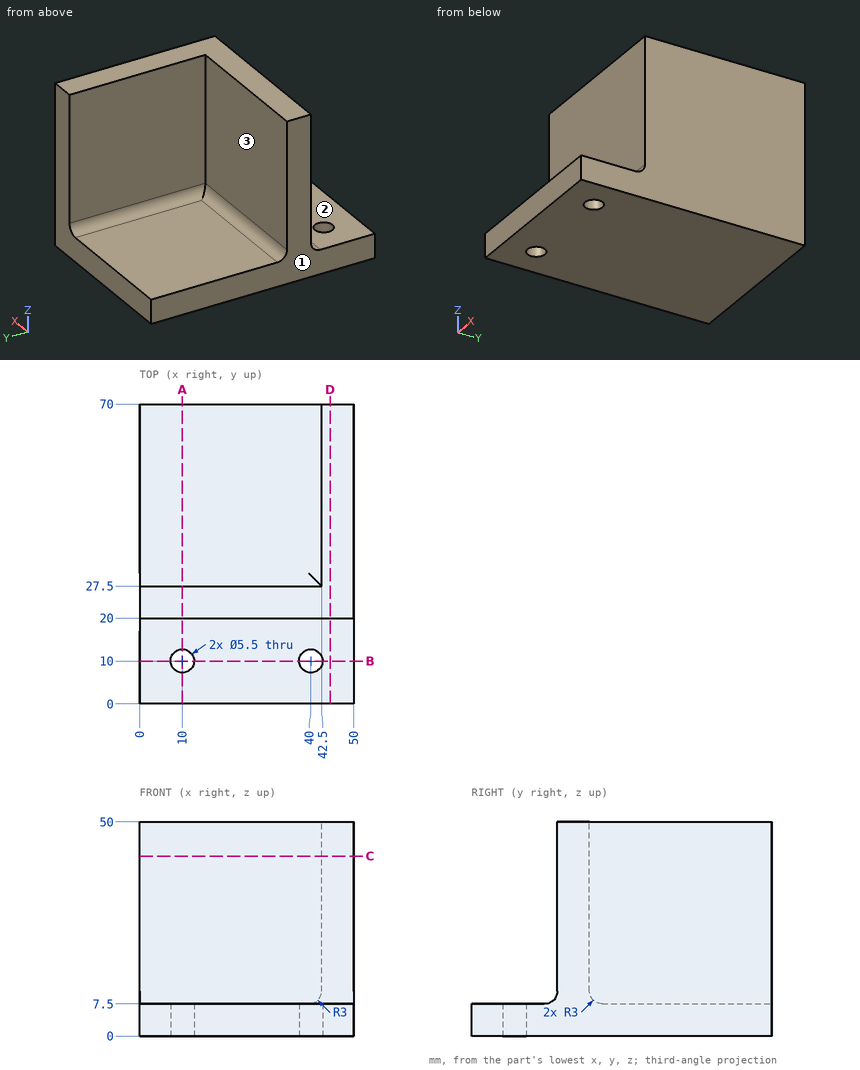
Geometry check sheet. Reference: drawing and pictorial views, mm from the part's lowest x, y, z. A direction names the side the tool comes from. Give positions to 0.01 mm unless a question says otherwise; leave off trailing zeros. Write each loop counter-clockwise with the first axis right and the second up, starting at its lowest first coordinate (ties: lowest second). Pieces come first, ordered by that corner, then holes. Notation, with made-up numbers: M 20.25,-3 L 75.25,-3 A5 cw 75.25,3 Z; hole C -2,59.25 d8. An arc over 180 degrees is marked long. Put each result on its own line as item: value. Start each with the question number.
1. Section check B-B (y = 10). Record the cut outline in (x, z).
2. Scan lines: line 1 along X through (y, z) = (10, 4.5); line 2 along Y through (x, z) = (10, 6.25); line 3 along Z through (x, y) = (17, 52). Record each from-to range of solid material in increasing order. Write a range as [from, to].
3. Go/stop test with flat-tipped pins: pin 1 Ø3 at (x, z) = (35, 27.5) entering from -Y; pin 2 Ø10 at (x, z) = (17, 30.5) entering from +Y; pin 3 Ø7 at (x, y) = (40, 10) entering from +Z. Record where each tip stops, or that it passes through.
4. Section check C-C (z = 42). Record the cut outline in (x, y).
5. Section check A-A (x = 10). Record the cut outline in (y, z), and give its area (3 significant figures).
6. Set-up check for the marked faces 1, 2 and 3: record each of +Z, -Z, +X, -X, +Y, -Y from which the full face is reachable in a straight line by a thin tool's end or side.
7. Section check D-D (x = 44.5). Record the cut outline in (y, z), and give its area (3 significant figures).
Answer list:
1. outline: M 0,0 L 7.25,0 L 7.25,7.5 L 0,7.5 Z; M 12.75,0 L 37.25,0 L 37.25,7.5 L 12.75,7.5 Z; M 42.75,0 L 50,0 L 50,7.5 L 42.75,7.5 Z
2. line 1: [0, 7.25], [12.75, 37.25], [42.75, 50]
2. line 2: [0, 7.25], [12.75, 70]
2. line 3: [0, 7.5]
3. pin 1: y = 20
3. pin 2: y = 27.5
3. pin 3: z = 7.5
4. outline: M 0,20 L 50,20 L 50,70 L 42.5,70 L 42.5,27.5 L 0,27.5 Z
5. outline: M 0,0 L 7.25,0 L 7.25,7.5 L 0,7.5 Z; M 12.75,0 L 70,0 L 70,7.5 L 30.5,7.5 A3 cw 27.5,10.5 L 27.5,50 L 20,50 L 20,10.5 A3 cw 17,7.5 L 12.75,7.5 Z
5. area: 806 mm2
6. face 1: +Z, -Z, -X, +Y, -Y
6. face 2: +Z, +X, -X, -Y
6. face 3: +Z, -X, +Y
7. outline: M 0,0 L 70,0 L 70,50 L 20,50 L 20,10.5 A3 cw 17,7.5 L 0,7.5 Z
7. area: 2,650 mm2
